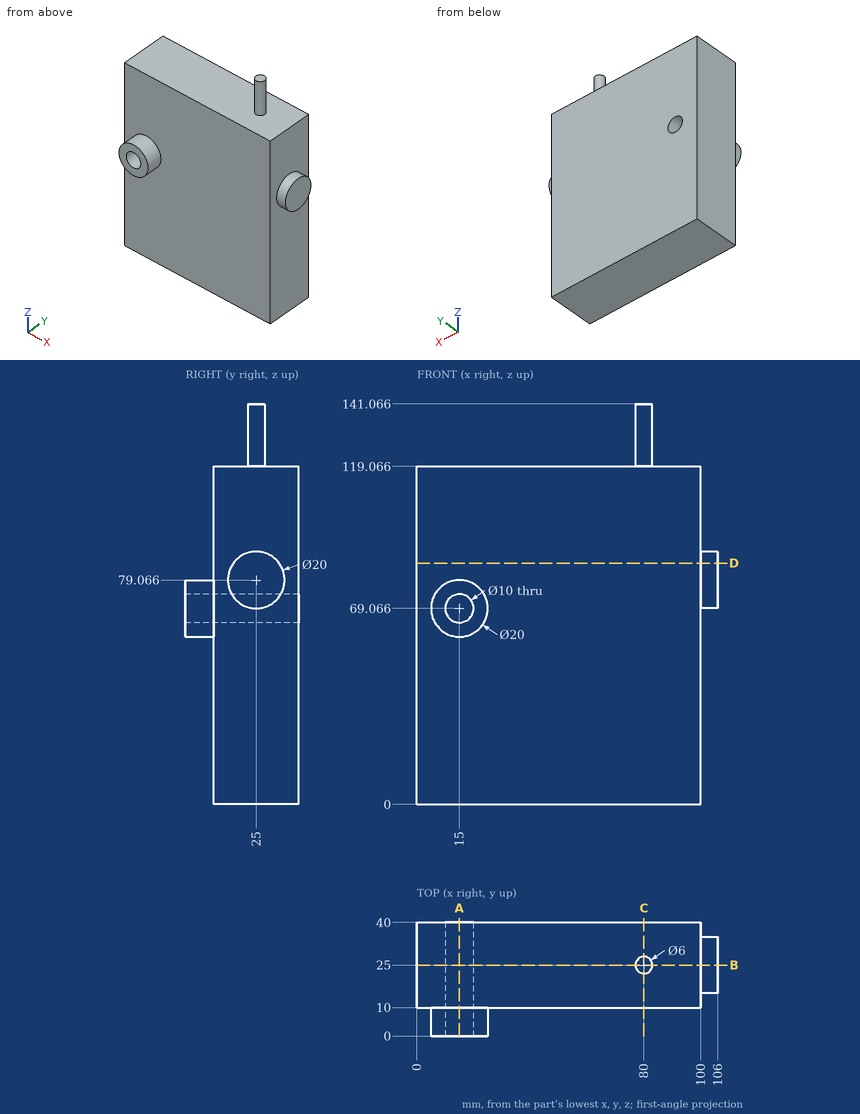
Answer from the drawing. Dimensions are ordinates in mm from the lowest x, y and z of the part. Give positions to 0.01 mm unless a question says otherwise; leave off trailing zeros. Loops run counter-clockwise (first coordinate to the right, second up) from the corner with the lowest first, then second, coordinate; pieces in that order, holes last. Notation, with made-up numbers: (82.25, 13) - (108.25, 13) arc R31 cw to (108.25, 47) - close; hole circle Ø8 at (7, 10). An arc over 180 degrees is marked (long way). Answer as CSV lines item,"result". Start each with the question number.
Item 1: A cutting plane is placed at D-D on z = 85. Determine the outline of the cut face in (x, y).
Item 2: A cutting plane is placed at B-B on y = 25. Determine the outline of the cut face in (x, z), then the cut area to 3 significant figures.
Item 3: Each of these flat-tipped pins is pushed along its axis until it touches: pin 1 (9 mm diameter, centred on x = 27, y = 20, fed in from +Z); pin 2 (5 mm diameter, centred on x = 40, z = 79.5, fed in from -Y); pin 3 (24 mm diameter, centred on y = 18.5, z = 30.5, fed in from +X). Where does it stop, or does it pass through?
Item 4: Find the intervals of material crossed by line 1 (Z direction, x = 15, y = 11); line 2 (X direction, y = 19.5, z = 38); line 3 (Z direction, x = 40.5, y = 36.5), in increasing order. Write a range as from..to.
Item 5: A cutting plane is placed at C-C on x = 80. Determine the outline of the cut face in (y, z), then the cut area to 3 significant figures.
Item 6: A cutting plane is placed at A-A on x = 15. Determine the outline of the cut face in (y, z), then the cut area to 3 significant figures.
Found:
1,outline,"(0, 10) - (100, 10) - (100, 16.95) - (106, 16.95) - (106, 33.05) - (100, 33.05) - (100, 40) - (0, 40) - close"
2,outline,"(0, 0) - (100, 0) - (100, 69.07) - (106, 69.07) - (106, 89.07) - (100, 89.07) - (100, 119.07) - (83, 119.07) - (83, 141.07) - (77, 141.07) - (77, 119.07) - (0, 119.07) - close; hole circle Ø10 at (15, 69.07)"
2,area,"12,100 mm^2"
3,pin 1,"stops at z = 119.07"
3,pin 2,"stops at y = 10"
3,pin 3,"stops at x = 100"
4,line 1,"z = 0..64.07, 74.07..119.07"
4,line 2,"x = 0..100"
4,line 3,"z = 0..119.07"
5,outline,"(10, 0) - (40, 0) - (40, 119.07) - (28, 119.07) - (28, 141.07) - (22, 141.07) - (22, 119.07) - (10, 119.07) - close"
5,area,"3,700 mm^2"
6,outline,"(0, 59.07) - (10, 59.07) - (10, 0) - (40, 0) - (40, 64.07) - (0, 64.07) - close; (0, 74.07) - (40, 74.07) - (40, 119.07) - (10, 119.07) - (10, 79.07) - (0, 79.07) - close"
6,area,"3,370 mm^2"
